```python
from build123d import *

# Parameters (mm, degrees)
F0_R      = 7.95
F1_DEPTH  = 3
F2_R      = 8.75
F3_DEPTH  = 3.5
F5_R      = 7.879792
F6_DEPTH  = 3
F7_R      = 1.77
F8_DEPTH  = 25
F9_R      = 6.858058
F9_R_2    = 2.485837
F9_R_3    = 0.921001
F10_DEPTH = 7


with BuildPart() as f1:
    # F0 (on Front) → F1 (new body)
    with BuildSketch(Plane.XZ):
        Circle(F0_R)
    extrude(amount=F1_DEPTH)

    # F2 (on face) → F3 (join)
    with BuildSketch(Plane(origin=(0, 0, 0), x_dir=(-1, 0, 0), z_dir=(0, 1, 0))):
        Circle(F2_R)
    extrude(amount=F3_DEPTH)

    # F5 (on face) → F6 (join)
    with BuildSketch(Plane(origin=(0, 3.5, 0), x_dir=(-1, 0, 0), z_dir=(0, 1, 0))):
        Circle(F5_R)
    extrude(amount=F6_DEPTH)

    # F7 (on face) → F8 (cut)
    with BuildSketch(Plane.XZ.offset(3)):
        with Locations((0, 5.088058)):
            Circle(F7_R)
        with Locations((-4.839031, 1.572297)):
            Circle(F7_R)
        with Locations((-2.990686, -4.116326)):
            Circle(F7_R)
        with Locations((2.990686, -4.116326)):
            Circle(F7_R)
        with Locations((4.839031, 1.572297)):
            Circle(F7_R)
    extrude(amount=-F8_DEPTH, mode=Mode.SUBTRACT)

    # F9 (on face) → F10 (cut)
    with BuildSketch(Plane.XZ.offset(3)):
        Circle(F9_R)
        Circle(F9_R_2, mode=Mode.SUBTRACT)
        Circle(F9_R_3)
    extrude(amount=-F10_DEPTH, mode=Mode.SUBTRACT)


solid = f1.part
```
Work out the finished part from the listing and answer in its coordinate system (mm). A direction names the side the tool comes from. Coordinates: 2 decimals unless noted, no trailing zeros. Write each loop counter-clockwise with the first axis right and the second up, starting at its lowest first coordinate (ties: lowest second). Pieces come first, ordered by that corner, then holes.
Q1. Find the intervals of material crossed by line 1 (Z direction, x = 0, y = 5.95); line 2 (Z direction, x = -2, y = 1.25); line 3 (Z direction, x = -0.25, y = 3), in increasing order.
Q2. A cutting plane is placed at B-B, the plane z = 3. Give the vertices of the cut face in (x, y), then the cut area to 3 significant figures.
Q3. Each of these flat-tipped pins is pushed along its axis until it touches: pin 1 Ø3 at (x, y) = (4, -1) entering from -Z; pin 2 Ø1 at (x, y) = (6, -1) entering from -Z; pin 3 Ø1.1 at (x, z) = (0, 0) entering from -Y. Where does it stop, or does it pass through?
Q4. A cutting plane is placed at C-C, the plane x = 2.75. Give the vertices of the cut face in (y, z).
Q5. A cutting plane is placed at D-D, the plane x = 4.5. Give the vertices of the cut face in (y, z), then the cut area to 3 significant figures.
Q6. Determine the mould class of faces 1 (the face through (6.944, 1.726, -5.324)), 2 (the face through (2.37, 0.45, 0.75)), 3 (the face through (0, -3, -1.1)) for opening direction Z: released by +Z, released by -Z, zero draft, split by the parting line, or undercut.
Q7. Which of the six approach directions +Z, -Z, +X, -X, +Y, -Y give full straight-line access (tool end or side, diameter ignored) to faces 4 (the face through (8, 3.5, 1)), 5 (the face through (0.121, 0.451, 6.857)), 6 (the face through (6.51, 5.25, 2.15))?
Q8. A cutting plane is placed at A-A, the plane y = -2. State how many separate pieces and enclosed holes the cut face has, then the cut area to 3 significant figures.
Findings below:
1. line 1: z = -7.88 to 3.32, 6.86 to 7.88
1. line 2: z = -8.52 to -6.56, -1.48 to 1.48, 6.56 to 8.52
1. line 3: z = -8.75 to -6.85, -2.47 to -0.89, 0.89 to 2.47, 6.85 to 8.75
2. outline: (-8.22, 0) - (-7.36, 0) - (-7.36, -3) - (-6.17, -3) - (-6.17, 4) - (-5.89, 4) - (-5.89, 6.5) - (-7.29, 6.5) - (-7.29, 3.5) - (-8.22, 3.5) - close; (-3.79, 4) - (3.79, 4) - (3.79, 6.5) - (-3.79, 6.5) - close; (5.89, 4) - (6.17, 4) - (6.17, -3) - (7.36, -3) - (7.36, 0) - (8.22, 0) - (8.22, 3.5) - (7.29, 3.5) - (7.29, 6.5) - (5.89, 6.5) - close
2. area: 48.6 mm2
3. pin 1: stops at z = -8.26
3. pin 2: stops at z = -5.74
3. pin 3: stops at y = 4
4. outline: (-3, -7.46) - (0, -7.46) - (0, -8.31) - (3.5, -8.31) - (3.5, -7.38) - (6.5, -7.38) - (6.5, -5.87) - (4, -5.87) - (4, -6.28) - (-3, -6.28) - close; (-3, 6.28) - (4, 6.28) - (4, -2.36) - (6.5, -2.36) - (6.5, 7.38) - (3.5, 7.38) - (3.5, 8.31) - (0, 8.31) - (0, 7.46) - (-3, 7.46) - close
5. outline: (-3, -6.55) - (0, -6.55) - (0, -7.5) - (3.5, -7.5) - (3.5, -6.47) - (6.5, -6.47) - (6.5, -5.04) - (4, -5.04) - (4, -5.18) - (-3, -5.18) - close; (-3, 5.18) - (4, 5.18) - (4, 3.31) - (6.5, 3.31) - (6.5, 6.47) - (3.5, 6.47) - (3.5, 7.5) - (0, 7.5) - (0, 6.55) - (-3, 6.55) - close; (4, -3.19) - (6.5, -3.19) - (6.5, -0.16) - (4, -0.16) - close
5. area: 44.9 mm2
6. face 1: split by the parting line
6. face 2: undercut
6. face 3: zero draft
7. face 4: +Y
7. face 5: -Y
7. face 6: +Y, -Y
8. separate pieces: 2
8. enclosed holes: 2
8. area: 67.5 mm2
